Read the model definition and answer for the solid it produces. Units are mm, in the model's axes. A direction names the side the tool comes from. Coordinates: 2 decimals unless noted, no trailing zeros. Write each loop counter-clockwise with the first axis right and the second up, starting at its lowest first coordinate (ties: lowest second). Pieces come first, ordered by that corner, then holes. Notation, with made-up numbers: (58, -23) -> (112, -23) arc R20 cw to (112, 1) -> close; hole circle Ø10 at (-36, -2.75). An arc over 180 degrees is marked (long way). Return JSON: item names as keys, results as strings.
from build123d import *

# Parameters (mm, degrees)
F0_W     = 1219.2
F0_H     = 88.9
F1_DEPTH = 19.05
F2_W     = 88.9
F2_H     = 609.6
F3_DEPTH = 88.9
F4_W     = 88.9
F4_H     = 609.6
F5_DEPTH = 88.9
F6_R     = 12.7
F7_DEPTH = 9.525
F8_R     = 25.4
F9_DEPTH = 6.35


with BuildPart() as f1:
    # F0 (on Top) → F1 (new body)
    with BuildSketch(Plane.XY):
        Rectangle(F0_W, F0_H)
    extrude(amount=F1_DEPTH)

    # F2 (on face) → F3 (join)
    with BuildSketch(Plane(origin=(0, 0, 0), x_dir=(1, 0, 0), z_dir=(0, 0, -1))):
        with Locations((-565.15, 0)):
            Rectangle(F2_W, F2_H)
    extrude(amount=F3_DEPTH)

    # F4 (on face) → F5 (join)
    with BuildSketch(Plane(origin=(0, 0, 0), x_dir=(1, 0, 0), z_dir=(0, 0, -1))):
        with Locations((565.15, 0)):
            Rectangle(F4_W, F4_H)
    extrude(amount=F5_DEPTH)

    # F6 (on face) → F7 (join)
    with BuildSketch(Plane(origin=(0, 0, -88.9), x_dir=(1, 0, 0), z_dir=(0, 0, -1))):
        with Locations((-565.15, 254)):
            Circle(F6_R)
        with Locations((-565.15, -254)):
            Circle(F6_R)
        with Locations((564.726949, 261.87405)):
            Circle(F6_R)
        with Locations((566.567481, -250.361617)):
            Circle(F6_R)
    extrude(amount=F7_DEPTH)

    # F8 (on face) → F9 (cut)
    with BuildSketch(Plane.XY):
        with BuildLine():
            ThreePointArc((-539.799658, -255.5875), (-539.762418, -254.794138), (-539.75, -254))
            ThreePointArc((-539.75, -254), (-539.762418, -253.205862), (-539.799658, -252.4125))
            ThreePointArc((-539.799658, -252.4125), (-590.55, -254), (-539.799658, -255.5875))
        make_face()
        with Locations((-565.15, 254)):
            Circle(F8_R)
        with Locations((565.15, 254)):
            Circle(F8_R)
        with Locations((565.15, -254)):
            Circle(F8_R)
        with BuildLine():
            ThreePointArc((-539.799658, -252.4125), (-539.762418, -253.205862), (-539.75, -254))
            ThreePointArc((-539.75, -254), (-539.762418, -254.794138), (-539.799658, -255.5875))
            Line((-539.799658, -255.5875), (-520.7, -255.5875))
            Line((-520.7, -255.5875), (-520.7, -254))
            Line((-520.7, -254), (-520.7, -252.4125))
            Line((-520.7, -252.4125), (-539.799658, -252.4125))
        make_face()
    extrude(amount=-F9_DEPTH, mode=Mode.SUBTRACT)


solid = f1.part
1. A tool of negligible diameter and unlimited length cuts with its end or side. For faces 1 (the face through (-7, 1, 0)), 2 (the face through (-564, -254, -6.35)), 3 (the face through (-566, 173, 0)), 4 (the face through (561.974, -249.476, -93.596)), 5 (the face through (565, -304.8, -44)), from which of +Z, -Z, +X, -X, +Y, -Y can it reach the whole face along a straight path? Write none if from no direction.
Taken from the geometry:
{"face 1": "-Z, +Y, -Y", "face 2": "+Z", "face 3": "+Z, +X, -X, +Y", "face 4": "-Z", "face 5": "+Z, -Z, +X, -X, -Y"}
2. Flat-ended cylindrical pins translate along their axes: pin 1 Ø15 at (x, y) = (559.5, -241.5) entering from +Z; pin 2 Ø1 at (x, y) = (-20.5, -20) entering from -Z; pin 3 Ø21 at (x, z) = (293.5, 9) entering from -Y. Find the tip coordinate at first contact, or state that the pin passes through.
Taken from the geometry:
{"pin 1": "stops at z = -6.35", "pin 2": "stops at z = 0", "pin 3": "stops at y = -44.45"}
3. The part is cut by section D-D (x = -244). Determine the outline of the cut face in (y, z), then the cut area to 3 significant figures.
Taken from the geometry:
{"outline": "(-44.45, 0) -> (44.45, 0) -> (44.45, 19.05) -> (-44.45, 19.05) -> close", "area": "1,690 mm2"}
4. Consider L1, parallel to Y at x = 565.15, z = -2.5; L2, parallel to X at y = 163.5, z = -58; L3, parallel to Z at x = -85, y = -36. Determine where each line is inside the solid, lowest interval first.
Taken from the geometry:
{"L1": "y = -304.8 to -279.4, -228.6 to 228.6, 279.4 to 304.8", "L2": "x = -609.6 to -520.7, 520.7 to 609.6", "L3": "z = 0 to 19.05"}
5. The part is cut by section C-C (x = 565.15). Determine the outline of the cut face in (y, z) (3 decimals), then the cut area to 3 significant figures.
Taken from the geometry:
{"outline": "(-304.8, -88.9) -> (-274.567, -88.9) -> (-274.567, -98.425) -> (-249.181, -98.425) -> (-249.181, -88.9) -> (237.741, -88.9) -> (237.741, -98.425) -> (262.982, -98.425) -> (262.982, -88.9) -> (304.8, -88.9) -> (304.8, 0) -> (279.4, 0) -> (279.4, -6.35) -> (228.6, -6.35) -> (228.6, 0) -> (44.45, 0) -> (44.45, 19.05) -> (-44.45, 19.05) -> (-44.45, 0) -> (-228.6, 0) -> (-228.6, -6.35) -> (-279.4, -6.35) -> (-279.4, 0) -> (-304.8, 0) -> close", "area": "55,700 mm2"}
6. The part is cut by section B-B (z = -41.5). Determine the outline of the cut face in (x, y), then the cut area to 3 significant figures.
Taken from the geometry:
{"outline": "(-609.6, -304.8) -> (-520.7, -304.8) -> (-520.7, 304.8) -> (-609.6, 304.8) -> close; (520.7, -304.8) -> (609.6, -304.8) -> (609.6, 304.8) -> (520.7, 304.8) -> close", "area": "108,000 mm2"}
7. The part is cut by section A-A (y = 93.5). Determine the outline of the cut face in (x, z).
Taken from the geometry:
{"outline": "(-609.6, -88.9) -> (-520.7, -88.9) -> (-520.7, 0) -> (-609.6, 0) -> close; (520.7, -88.9) -> (609.6, -88.9) -> (609.6, 0) -> (520.7, 0) -> close"}
